```python
from build123d import *

# Parameters (mm, degrees)
F0_W     = 26
F0_H     = 61
F1_DEPTH = 6


with BuildPart() as f1:
    # F0 (on Front) → F1 (new body)
    with BuildSketch(Plane.XZ):
        Polygon((-231.5, -176.5), (223.5, -176.5), (243.5, -176.5), (243.5, -156.5), (243.5, 148.5), (243.5, 168.5), (227.5, 168.5), (-227.5, 168.5), (-251.5, 168.5), (-251.5, 152.5), (-251.5, -152.5), (-251.5, -176.5), align=None)
        with Locations((-215.17, -126.66)):
            Rectangle(F0_W, F0_H, mode=Mode.SUBTRACT)
        with Locations((-170.84, -126.66)):
            Rectangle(F0_W, F0_H, mode=Mode.SUBTRACT)
        with Locations((-126.51, -126.66)):
            Rectangle(F0_W, F0_H, mode=Mode.SUBTRACT)
        with Locations((-82.18, -126.66)):
            Rectangle(F0_W, F0_H, mode=Mode.SUBTRACT)
        with Locations((-37.85, -126.66)):
            Rectangle(F0_W, F0_H, mode=Mode.SUBTRACT)
        with Locations((-215.17, -51.33)):
            Rectangle(F0_W, F0_H, mode=Mode.SUBTRACT)
        with Locations((-170.84, -51.33)):
            Rectangle(F0_W, F0_H, mode=Mode.SUBTRACT)
        with Locations((-126.51, -51.33)):
            Rectangle(F0_W, F0_H, mode=Mode.SUBTRACT)
        with Locations((-82.18, -51.33)):
            Rectangle(F0_W, F0_H, mode=Mode.SUBTRACT)
        with Locations((-37.85, -51.33)):
            Rectangle(F0_W, F0_H, mode=Mode.SUBTRACT)
        with Locations((29.83, -126.66)):
            Rectangle(F0_W, F0_H, mode=Mode.SUBTRACT)
        with Locations((74.16, -126.66)):
            Rectangle(F0_W, F0_H, mode=Mode.SUBTRACT)
        with Locations((118.49, -126.66)):
            Rectangle(F0_W, F0_H, mode=Mode.SUBTRACT)
        with Locations((162.82, -126.66)):
            Rectangle(F0_W, F0_H, mode=Mode.SUBTRACT)
        with Locations((207.15, -126.66)):
            Rectangle(F0_W, F0_H, mode=Mode.SUBTRACT)
        with Locations((29.83, -51.33)):
            Rectangle(F0_W, F0_H, mode=Mode.SUBTRACT)
        with Locations((74.16, -51.33)):
            Rectangle(F0_W, F0_H, mode=Mode.SUBTRACT)
        with Locations((118.49, -51.33)):
            Rectangle(F0_W, F0_H, mode=Mode.SUBTRACT)
        with Locations((162.82, -51.33)):
            Rectangle(F0_W, F0_H, mode=Mode.SUBTRACT)
        with Locations((207.15, -51.33)):
            Rectangle(F0_W, F0_H, mode=Mode.SUBTRACT)
        with Locations((-215.17, 43.34)):
            Rectangle(F0_W, F0_H, mode=Mode.SUBTRACT)
        with Locations((-170.84, 43.34)):
            Rectangle(F0_W, F0_H, mode=Mode.SUBTRACT)
        with Locations((-126.51, 43.34)):
            Rectangle(F0_W, F0_H, mode=Mode.SUBTRACT)
        with Locations((-82.18, 43.34)):
            Rectangle(F0_W, F0_H, mode=Mode.SUBTRACT)
        with Locations((-37.85, 43.34)):
            Rectangle(F0_W, F0_H, mode=Mode.SUBTRACT)
        with Locations((-215.17, 118.67)):
            Rectangle(F0_W, F0_H, mode=Mode.SUBTRACT)
        with Locations((-170.84, 118.67)):
            Rectangle(F0_W, F0_H, mode=Mode.SUBTRACT)
        with Locations((-126.51, 118.67)):
            Rectangle(F0_W, F0_H, mode=Mode.SUBTRACT)
        with Locations((-82.18, 118.67)):
            Rectangle(F0_W, F0_H, mode=Mode.SUBTRACT)
        with Locations((-37.85, 118.67)):
            Rectangle(F0_W, F0_H, mode=Mode.SUBTRACT)
        with Locations((29.83, 43.34)):
            Rectangle(F0_W, F0_H, mode=Mode.SUBTRACT)
        with Locations((74.16, 43.34)):
            Rectangle(F0_W, F0_H, mode=Mode.SUBTRACT)
        with Locations((118.49, 43.34)):
            Rectangle(F0_W, F0_H, mode=Mode.SUBTRACT)
        with Locations((162.82, 43.34)):
            Rectangle(F0_W, F0_H, mode=Mode.SUBTRACT)
        with Locations((207.15, 43.34)):
            Rectangle(F0_W, F0_H, mode=Mode.SUBTRACT)
        with Locations((29.83, 118.67)):
            Rectangle(F0_W, F0_H, mode=Mode.SUBTRACT)
        with Locations((74.16, 118.67)):
            Rectangle(F0_W, F0_H, mode=Mode.SUBTRACT)
        with Locations((118.49, 118.67)):
            Rectangle(F0_W, F0_H, mode=Mode.SUBTRACT)
        with Locations((162.82, 118.67)):
            Rectangle(F0_W, F0_H, mode=Mode.SUBTRACT)
        with Locations((207.15, 118.67)):
            Rectangle(F0_W, F0_H, mode=Mode.SUBTRACT)
    extrude(amount=F1_DEPTH)


solid = f1.part
```
Design review of the part built by this model. Coordinates are the model's own, in mm. Coordinates: 2 decimals unless noted, no trailing zeros. Write each loop counter-clockwise with the first axis right and the second up, starting at its lowest first coordinate (ties: lowest second). Pieces come first, ordered by that corner, then holes.
1) Insertion check: pin 1 (12 mm diameter, centred on x = 140, z = -65.5, fed in from +Y). The pin has a flat end and moves straight along its axis. Give the tip position at first contact, or say it passes through.
2) To check wall thickness, follow L1, parallel to Z at x = -115.5, y = -1.55. State the ranges of the line that lie inside material, in increasing order.
3) Add section A-A (x = 30.5). Write out the cut boundary in (y, z).
4) Add section B-B (y = -1.15). State how many separate pieces and enclosed holes the cut face has, plus the area to 3 significant figures.
Check result:
1. pin 1: stops at y = 0
2. L1: z = -176.5 to -157.16, -96.16 to -81.83, -20.83 to 12.84, 73.84 to 88.17, 149.17 to 168.5
3. outline: (-6, -176.5) - (0, -176.5) - (0, -157.16) - (-6, -157.16) - close; (-6, -96.16) - (0, -96.16) - (0, -81.83) - (-6, -81.83) - close; (-6, -20.83) - (0, -20.83) - (0, 12.84) - (-6, 12.84) - close; (-6, 73.84) - (0, 73.84) - (0, 88.17) - (-6, 88.17) - close; (-6, 149.17) - (0, 149.17) - (0, 168.5) - (-6, 168.5) - close
4. separate pieces: 1
4. enclosed holes: 40
4. area: 107,000 mm2
